Check sheet for the drawn part. Datum: minimum x, y, z corner. Units: mm. A direction names the side the tool comes from. Coordinates: 2 decimals unless noted, no trailing zeros. Loops run counter-clockwise (first coordinate to the right, second up) from the corner with the lowest first, then second, coordinate; pieces in that order, holes last.
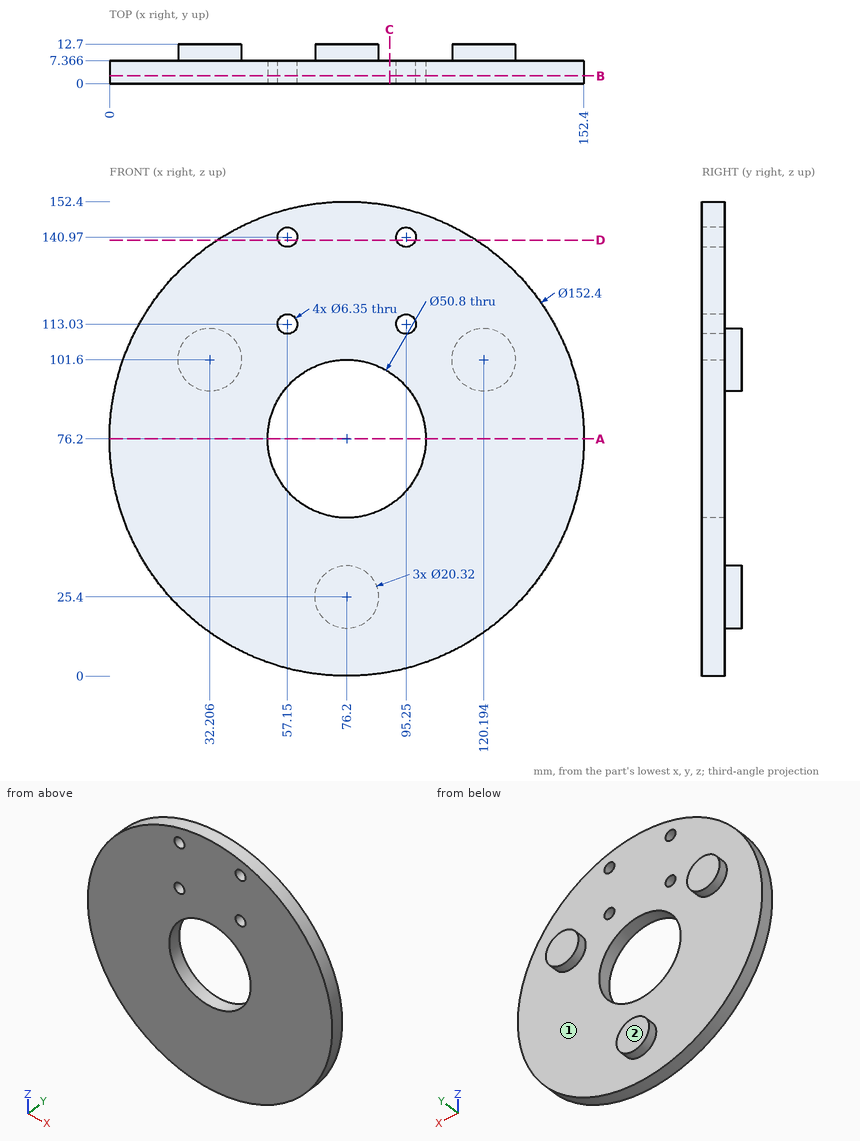
1) Section check B-B on y = 2.5. Enter the section's corners in (x, z) (3 decimals).
Answer sheet:
outline: circle Ø152.4 at (76.2, 76.2); hole circle Ø50.8 at (76.2, 76.2); hole circle Ø6.35 at (57.15, 113.03); hole circle Ø6.35 at (57.15, 140.97); hole circle Ø6.35 at (95.25, 113.03); hole circle Ø6.35 at (95.25, 140.97)
2) Section check D-D on z = 140. Enter the section's corners in (x, y).
Answer sheet:
outline: (34.53, 0) - (54.13, 0) - (54.13, 7.37) - (34.53, 7.37) - close; (60.17, 0) - (92.23, 0) - (92.23, 7.37) - (60.17, 7.37) - close; (98.27, 0) - (117.87, 0) - (117.87, 7.37) - (98.27, 7.37) - close
3) Section check A-A on z = 76.2. Enter the section's corners in (x, y).
Answer sheet:
outline: (0, 0) - (50.8, 0) - (50.8, 7.37) - (0, 7.37) - close; (101.6, 0) - (152.4, 0) - (152.4, 7.37) - (101.6, 7.37) - close
4) Depth check by flat-ended pin: pin 1 (5 mm diameter, centred on x = 57.15, z = 140.97, fed in from -Y); pin 2 (2 mm diameter, centred on y = 1.5, z = 41.5, fed in from +X); pin 3 (1.5 mm diameter, centred on y = 3.5, z = 25.5, fed in from +X) (3 decimals); pin 4 (2 mm diameter, centred on x = 106, y = 7, fed in from +Z). Enter the tip coordinate at first touch or a pass-through.
Answer sheet:
pin 1: passes through
pin 2: stops at x = 144.54
pin 3: stops at x = 133.745
pin 4: stops at z = 146.75
5) Scan lines: line 1 (X direction, y = 3.25, z = 140.97) (1 decimal); line 2 (X direction, y = 4.5, z = 75); line 3 (X direction, y = 5, z = 113.03) (1 decimal). Record each from-to range of solid material in increasing order.
Answer sheet:
line 1: x = 36.1 to 54, 60.3 to 92.1, 98.4 to 116.3
line 2: x = 0.01 to 50.83, 101.57 to 152.39
line 3: x = 9.5 to 54, 60.3 to 92.1, 98.4 to 142.9
6) Section check C-C on x = 90. Enter the section's corners in (y, z).
Answer sheet:
outline: (0, 1.26) - (7.37, 1.26) - (7.37, 54.88) - (0, 54.88) - close; (0, 97.52) - (7.37, 97.52) - (7.37, 151.14) - (0, 151.14) - close
7) Set-up check for the marked faces 1 and 2: record each of +Z, -Z, +X, -X, +Y, -Y from which the full face is reachable in a straight line by a thin tool's end or side.
Answer sheet:
face 1: +Y
face 2: +Z, -Z, +X, -X, +Y
